```python
from build123d import *

# Parameters (mm, degrees)
SKETCH1_R           = 46.99
SKETCH1_R_2         = 8.509
SKETCH1_R_3         = 4
BOSS_EXTRUDE1_DEPTH = 10
BOSS_EXTRUDE2_DEPTH = 90
SKETCH4_R           = 10
BOSS_EXTRUDE3_DEPTH = 10
FILLET2_R           = 20


with BuildPart() as part:
    # Sketch1 → Boss-Extrude1 (new body)
    # profile 1 of 2: a face of its own
    with BuildSketch(Plane(origin=(0, 0, 0), x_dir=(1, 0, 0), z_dir=(0, 1, 0))):
        with Locations(Location((0, 0, 0), (0, 0, 270))):
            Circle(SKETCH1_R)
        Circle(SKETCH1_R_2, mode=Mode.SUBTRACT)
        with Locations(Location((-32.475952642, 18.75, 0), (0, 0, 270))):
            Circle(SKETCH1_R_3, mode=Mode.SUBTRACT)
        with Locations(Location((-32.475952642, -18.75, 0), (0, 0, 270))):
            Circle(SKETCH1_R_3, mode=Mode.SUBTRACT)
        with Locations(Location((0, -37.5, 0), (0, 0, 270))):
            Circle(SKETCH1_R_3, mode=Mode.SUBTRACT)
        with Locations(Location((32.475952642, -18.75, 0), (0, 0, 270))):
            Circle(SKETCH1_R_3, mode=Mode.SUBTRACT)
        with Locations(Location((32.475952642, 18.75, 0), (0, 0, 270))):
            Circle(SKETCH1_R_3, mode=Mode.SUBTRACT)
        with Locations(Location((0, 37.5, 0), (0, 0, 270))):
            Circle(SKETCH1_R_3, mode=Mode.SUBTRACT)
    # profile 2 of 2: a face of its own
    with BuildSketch(Plane(origin=(0, 0, 0), x_dir=(1, 0, 0), z_dir=(0, 1, 0))):
        Circle(SKETCH1_R_2)
    extrude(amount=BOSS_EXTRUDE1_DEPTH)

    # Sketch2 → Boss-Extrude2 (add)
    with BuildSketch(Plane(origin=(0, 10, 0), x_dir=(1, 0, 0), z_dir=(0, 1, 0))):
        with BuildLine():
            Line((-5.708203932, 5.605034154), (-7.485281374, 6.631030293))
            ThreePointArc((-7.485281374, 6.631030293), (-8.660254038, 5), (-9.485281374, 3.166928678))
            Line((-9.485281374, 3.166928678), (-7.708203932, 2.140932539))
            ThreePointArc((-7.708203932, 2.140932539), (-8, 0), (-7.708203932, -2.140932539))
            Line((-7.708203932, -2.140932539), (-9.485281374, -3.166928678))
            ThreePointArc((-9.485281374, -3.166928678), (-8.660254038, -5), (-7.485281374, -6.631030293))
            Line((-7.485281374, -6.631030293), (-5.708203932, -5.605034154))
            ThreePointArc((-5.708203932, -5.605034154), (-4, -6.92820323), (-2, -7.745966692))
            Line((-2, -7.745966692), (-2, -9.797958971))
            ThreePointArc((-2, -9.797958971), (0, -10), (2, -9.797958971))
            Line((2, -9.797958971), (2, -7.745966692))
            ThreePointArc((2, -7.745966692), (4, -6.92820323), (5.708203932, -5.605034154))
            Line((5.708203932, -5.605034154), (7.485281374, -6.631030293))
            ThreePointArc((7.485281374, -6.631030293), (8.660254038, -5), (9.485281374, -3.166928678))
            Line((9.485281374, -3.166928678), (7.708203932, -2.140932539))
            ThreePointArc((7.708203932, -2.140932539), (8, 0), (7.708203932, 2.140932539))
            Line((7.708203932, 2.140932539), (9.485281374, 3.166928678))
            ThreePointArc((9.485281374, 3.166928678), (8.660254038, 5), (7.485281374, 6.631030293))
            Line((7.485281374, 6.631030293), (5.708203932, 5.605034154))
            ThreePointArc((5.708203932, 5.605034154), (4, 6.92820323), (2, 7.745966692))
            Line((2, 7.745966692), (2, 9.797958971))
            ThreePointArc((2, 9.797958971), (0, 10), (-2, 9.797958971))
            Line((-2, 9.797958971), (-2, 7.745966692))
            ThreePointArc((-2, 7.745966692), (-4, 6.92820323), (-5.708203932, 5.605034154))
        make_face()
    extrude(amount=BOSS_EXTRUDE2_DEPTH)

    # Sketch4 → Boss-Extrude3 (add)
    with BuildSketch(Plane(origin=(0, 10, 0), x_dir=(1, 0, 0), z_dir=(0, 1, 0))):
        with Locations(Location((0, 0, 0), (0, 0, 101.536959033))):
            Circle(SKETCH4_R)
    extrude(amount=BOSS_EXTRUDE3_DEPTH)

    # Fillet2
    # the kernel refuses this fillet: 20 mm, written as the material it adds along each edge
    with BuildSketch(Plane(origin=(0, 20, 0), x_dir=(0.9893271243483546, 0, 0.1457114993012412), z_dir=(0.1457114993012412, 0, -0.9893271243483546))) as fillet2_piece_1:
        with BuildLine():
            CenterArc((28, -8.717797887), FILLET2_R, 154.158067237, 25.841932763)
            Line((8, -8.717797887), (8, 0))
            Line((8, 0), (10, 0))
        make_face()
    revolve(axis=Axis((0, 20, 0), (0, -1, 0)), revolution_arc=343.243034599)
    with BuildSketch(Plane(origin=(0, 20, 0), x_dir=(0.6208534221926202, 0, -0.7839266726880214), z_dir=(-0.7839266726880214, 0, -0.6208534221926202))) as fillet2_piece_2:
        with BuildLine():
            CenterArc((28, -8.717797887), FILLET2_R, 154.158067237, 25.841932763)
            Line((8, -8.717797887), (8, 0))
            Line((8, 0), (10, 0))
        make_face()
    revolve(axis=Axis((0, 20, 0), (0, -1, 0)), revolution_arc=343.243034599)
    with BuildSketch(Plane(origin=(0, 20, 0), x_dir=(-0.36847370215574865, 0, -0.9296381719893158), z_dir=(-0.9296381719893158, 0, 0.36847370215574865))) as fillet2_piece_3:
        with BuildLine():
            CenterArc((28, -8.717797887), FILLET2_R, 154.158067237, 25.841932763)
            Line((10, 0), (8, 0))
            Line((8, 0), (8, -8.717797887))
        make_face()
    revolve(axis=Axis((0, 20, 0), (0, -1, 0)), revolution_arc=343.243034599)
    with BuildSketch(Plane(origin=(0, 20, 0), x_dir=(-0.9893271243483555, 0, -0.14571149930123434), z_dir=(-0.14571149930123434, 0, 0.9893271243483555))) as fillet2_piece_4:
        with BuildLine():
            CenterArc((28, -8.717797887), FILLET2_R, 154.158067237, 25.841932763)
            Line((10, 0), (8, 0))
            Line((8, 0), (8, -8.717797887))
        make_face()
    revolve(axis=Axis((0, 20, 0), (0, -1, 0)), revolution_arc=343.243034599)
    with BuildSketch(Plane(origin=(0, 20, 0), x_dir=(-0.6208534221925923, 0, 0.7839266726880435), z_dir=(0.7839266726880435, 0, 0.6208534221925923))) as fillet2_piece_5:
        with BuildLine():
            CenterArc((28, -8.717797887), FILLET2_R, 154.158067237, 25.841932763)
            Line((8, -8.717797887), (8, 0))
            Line((8, 0), (10, 0))
        make_face()
    revolve(axis=Axis((0, 20, 0), (0, -1, 0)), revolution_arc=343.243034599)
    with BuildSketch(Plane(origin=(0, 20, 0), x_dir=(0.3684737021557518, 0, 0.9296381719893145), z_dir=(0.9296381719893145, 0, -0.3684737021557518))) as fillet2_piece_6:
        with BuildLine():
            CenterArc((28, -8.717797887), FILLET2_R, 154.158067237, 25.841932763)
            Line((8, -8.717797887), (8, 0))
            Line((8, 0), (10, 0))
        make_face()
    revolve(axis=Axis((0, 20, 0), (0, -1, 0)), revolution_arc=343.243034599)

    # Sketch7 → Cut-Revolve1 (revolve, cut)
    with BuildSketch(Plane(origin=(0, 0, 0), x_dir=(0, 0, -1), z_dir=(1, 0, 0)), mode=Mode.PRIVATE) as cut_revolve1_sk:
        Polygon((10, 100), (10, 96.535898385), (8, 100), align=None)
    revolve(cut_revolve1_sk.sketch.rotate(Axis((0, 136.433969782, 0), (0, -1, 0)), 348.463040967), axis=Axis((0, 136.433969782, 0), (0, -1, 0)), mode=Mode.SUBTRACT)


solid = part.part
```
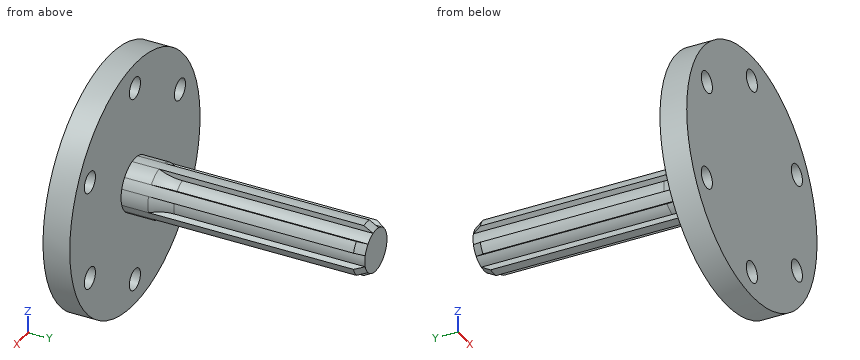
Source: CAD feature listing. Evaluate the final solid. Frame: model axes, mm. Give positions to 0.01 mm unless a question says otherwise; leave off trailing zeros. Loops run counter-clockwise (first coordinate to the right, second up) from the corner with the lowest first, then second, coordinate; pieces in that order, holes last. Notation, with made-up numbers: M 53.25,12.25 L 99.25,12.25 A21 cw 99.25,50.25 Z; hole C 63,67 d8. An arc over 180 degrees is marked long. Put each result on its own line as item: value.
Q1. Section B-B (y = 41). Return the cut outline in (x, z).
Response values:
outline: M -9.49,-3.17 A10 ccw -7.49,-6.63 L -5.71,-5.61 A8 ccw -2,-7.75 L -2,-9.8 A10 ccw 2,-9.8 L 2,-7.75 A8 ccw 5.71,-5.61 L 7.49,-6.63 A10 ccw 9.49,-3.17 L 7.71,-2.14 A8 ccw 7.71,2.14 L 9.49,3.17 A10 ccw 7.49,6.63 L 5.71,5.61 A8 ccw 2,7.75 L 2,9.8 A10 ccw -2,9.8 L -2,7.75 A8 ccw -5.71,5.61 L -7.49,6.63 A10 ccw -9.49,3.17 L -7.71,2.14 A8 ccw -7.71,-2.14 Z
Q2. Section C-C (z = 37.5). Return the cut outline in (x, y).
Response values:
outline: M -28.32,0 L -4,0 L -4,10 L -28.32,10 Z; M 4,0 L 28.32,0 L 28.32,10 L 4,10 Z
Q3. Pin query (flat end, axial travel): P1, Ø6.5, axis at x = 32.48, z = -18.75, coming from the +Y side; P2, Ø5, axis at y = 86.5, z = -3, coming from the +X side; P3, Ø1, axis at y = 40.5, z = -8.5, coming from the -X side; P4, Ø10, axis at x = -9, y = 48, coming from the -Z side. Return the tip coordinate at first contact, or that it passes through.
Response values:
P1: passes through
P2: stops at x = 9.49
P3: stops at x = -2
P4: stops at z = -6.93
Q4. Section A-A (z = -18.75). Return the cut outline in (x, y).
Response values:
outline: M -43.09,0 L -36.48,0 L -36.48,10 L -43.09,10 Z; M -28.48,0 L 28.48,0 L 28.48,10 L -28.48,10 Z; M 36.48,0 L 43.09,0 L 43.09,10 L 36.48,10 Z
Q5. Line query: probe 1 along X at (y, z) = (4, -18); probe 2 along Z at (x, y) = (0, 60.5); probe 3 along X at (y, z) = (63, 2). Output: solid intervals per line, ascending. Write a range as [from, to].
Response values:
probe 1: x = [-43.41, -36.41], [-28.55, 28.55], [36.41, 43.41]
probe 2: z = [-10, 10]
probe 3: x = [-7.75, 7.75]
Q6. Section D-D (z = 0). Return the cut outline in (x, y).
Response values:
outline: M -46.99,0 L 46.99,0 L 46.99,10 L 10,10 L 10,20 A20 cw 8,28.72 L 8,100 L -8,100 L -8,28.72 A20 cw -10,20 L -10,10 L -46.99,10 Z
